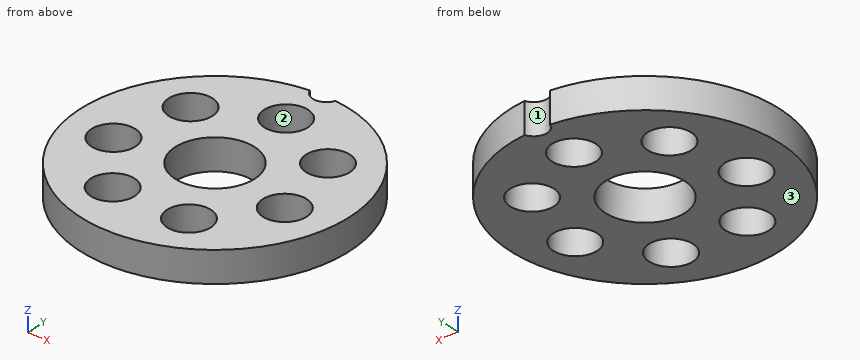
```python
from build123d import *

# Parameters (mm, degrees)
SKETCH1_R           = 1.7272
SKETCH1_R_2         = 3.1242
BOSS_EXTRUDE1_DEPTH = 2.4384


with BuildPart() as part:
    # Sketch1 → Boss-Extrude1 (new body)
    with BuildSketch(Plane.XY):
        with BuildLine():
            ThreePointArc((-1.0033, 10.544174522), (0, -10.5918), (1.0033, 10.544174522))
            ThreePointArc((1.0033, 10.544174522), (0, 9.8298), (-1.0033, 10.544174522))
        make_face()
        with Locations((0, 6.9596)):
            Circle(SKETCH1_R, mode=Mode.SUBTRACT)
        with Locations((-5.441234385, 4.339239625)):
            Circle(SKETCH1_R, mode=Mode.SUBTRACT)
        with Locations((-6.785108298, -1.548656692)):
            Circle(SKETCH1_R, mode=Mode.SUBTRACT)
        with Locations((-3.019657271, -6.270382933)):
            Circle(SKETCH1_R, mode=Mode.SUBTRACT)
        with Locations((3.019657271, -6.270382933)):
            Circle(SKETCH1_R, mode=Mode.SUBTRACT)
        with Locations((6.785108298, -1.548656692)):
            Circle(SKETCH1_R, mode=Mode.SUBTRACT)
        with Locations((5.441234385, 4.339239625)):
            Circle(SKETCH1_R, mode=Mode.SUBTRACT)
        Circle(SKETCH1_R_2, mode=Mode.SUBTRACT)
    extrude(amount=BOSS_EXTRUDE1_DEPTH)


solid = part.part
```
Check sheet for the modelled part. Datum: model origin and axes. Units: mm. Face numbers are marked on the shaded views. Round coordinates to 2 decimals unless told otherwise and drop trailing zeros. Loops run counter-clockwise (first coordinate to the right, second up) from the corner with the lowest first, then second, coordinate; pieces in that order, holes last. Notation, with made-up numbers: (45, 65) -> (65, 65) arc R11 cw to (65, 73) -> close; hole circle Ø5 at (45, -22.75). An arc over 180 degrees is marked (long way). Write item = value, one per line. Start each with the question number.
1) Sectioned sample at A-A, the plane x = 0. Record the cut outline in (y, z), plus the area to 3 significant figures.
2) Sectioned sample at B-B, the plane y = 4. Record the cut outline in (x, z), plus the area to 3 significant figures.
3) Thickness scan on probe 1 along X at (y, z) = (-1, 1.3); probe 2 along X at (y, z) = (-5.25, 0.6); probe 3 along X at (y, z) = (5.5, 0.8). Record the ranges inside material, lowest first.
4) Release check for a two-part mould opening along Y. For the marked faces 1, 2 and 3 record: released by +Y, released by -Y, zero draft, split by the parting line, or undercut.
5) Sectioned sample at D-D, the plane z = 1.7. State how many separate pieces and enclosed holes the cut face has, plus the area to 3 significant figures.
6) Sectioned sample at C-C, the plane x = 8. Record the cut outline in (y, z), plus the area to 3 significant figures.
Results are:
q1.outline = (-10.59, 0) -> (-3.12, 0) -> (-3.12, 2.44) -> (-10.59, 2.44) -> close; (3.12, 0) -> (5.23, 0) -> (5.23, 2.44) -> (3.12, 2.44) -> close; (8.69, 0) -> (9.83, 0) -> (9.83, 2.44) -> (8.69, 2.44) -> close
q1.area = 26.1 mm^2
q2.outline = (-9.81, 0) -> (-7.13, 0) -> (-7.13, 2.44) -> (-9.81, 2.44) -> close; (-3.75, 0) -> (3.75, 0) -> (3.75, 2.44) -> (-3.75, 2.44) -> close; (7.13, 0) -> (9.81, 0) -> (9.81, 2.44) -> (7.13, 2.44) -> close
q2.area = 31.3 mm^2
q3.probe_1 = -10.54 to -8.42, -5.15 to -2.96, 2.96 to 5.15, 8.42 to 10.54
q3.probe_2 = -9.2 to -4.41, -1.63 to 1.63, 4.41 to 9.2
q3.probe_3 = -9.05 to -6.72, -4.16 to -0.92, 0.92 to 4.16, 6.72 to 9.05
q4.face_1 = released by +Y
q4.face_2 = undercut
q4.face_3 = zero draft
q5.separate_pieces = 1
q5.enclosed_holes = 8
q5.area = 255 mm^2
q6.outline = (-6.94, 0) -> (-2.78, 0) -> (-2.78, 2.44) -> (-6.94, 2.44) -> close; (-0.32, 0) -> (6.94, 0) -> (6.94, 2.44) -> (-0.32, 2.44) -> close
q6.area = 27.9 mm^2
